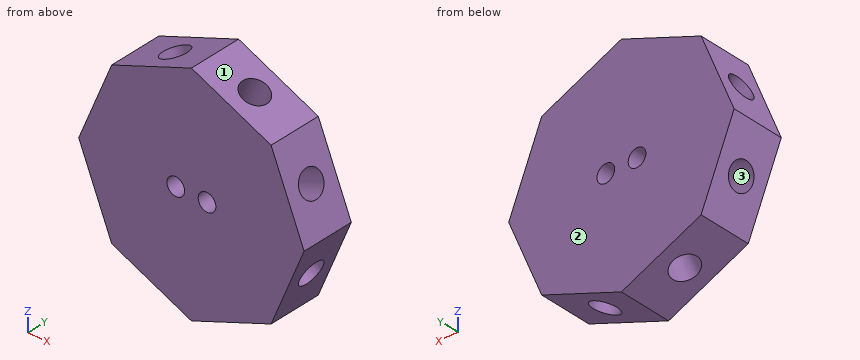
from build123d import *

# Parameters (mm, degrees)
SKETCH1_R           = 1.0795
BOSS_EXTRUDE1_DEPTH = 6.35
SKETCH2_R           = 1.5875
CUT_EXTRUDE1_DEPTH  = 7.62
CIRPATTERN1_COUNT   = 8


with BuildPart() as part:
    # Sketch1 → Boss-Extrude1 (new body)
    with BuildSketch(Plane(origin=(0, 0, 0), x_dir=(1, 0, 0), z_dir=(0, 1, 0))):
        Polygon((0, 13.746380944), (-9.720159182, 9.720159182), (-13.746380944, 0), (-9.720159182, -9.720159182), (0, -13.746380944), (9.720159182, -9.720159182), (13.746380944, 0), (9.720159182, 9.720159182), align=None)
        with Locations(Location((1.905, 0, 0), (0, 0, 270))):
            Circle(SKETCH1_R, mode=Mode.SUBTRACT)
        with Locations(Location((-1.905, 0, 0), (0, 0, 270))):
            Circle(SKETCH1_R, mode=Mode.SUBTRACT)
    extrude(amount=BOSS_EXTRUDE1_DEPTH)

    # Sketch2 → Cut-Extrude1 (cut)
    with BuildSketch(Plane(origin=(-4.860079591, 0, 11.733270063), x_dir=(0.9238795325112905, 0, 0.3826834323650806), z_dir=(-0.3826834323650806, 0, 0.9238795325112905))):
        with Locations((0, 3.175)):
            Circle(SKETCH2_R)
    cut_extrude1 = extrude(amount=-CUT_EXTRUDE1_DEPTH, mode=Mode.SUBTRACT)

    # CirPattern1: Cut-Extrude1 ×8 about axis
    cirpattern1_axis = Axis((0, 0, 0), (0, 1, 0))
    for i in range(1, CIRPATTERN1_COUNT):
        add(cut_extrude1.rotate(cirpattern1_axis, i * 360 / CIRPATTERN1_COUNT), mode=Mode.SUBTRACT)


solid = part.part
Verification items for the finished model (mm, model axes). Face numbers are marked on the shaded views. Coordinates: 2 decimals unless noted, no trailing zeros. Loops run counter-clockwise (first coordinate to the right, second up) from the corner with the lowest first, then second, coordinate; pieces in that order, holes last. Notation, with made-up numbers: (-28, -37.5) -> (13, -37.5) arc R22 cw to (13, -7.5) -> close; hole circle Ø6 at (39.25, -12.75). An arc over 180 degrees is marked (long way). Answer as a JSON object with one key per item and string values. Group by question number.
Item 1: Depth check by flat-ended pin: pin 1 (1 mm diameter, centred on x = 6.5, y = 3, fed in from -Z); pin 2 (3 mm diameter, centred on x = -1.905, z = 0, fed in from -Y); pin 3 (2 mm diameter, centred on x = 2, y = 1.5, fed in from -Z). Enter the tip coordinate at first touch or a pass-through.
Item 2: Mould release check, pull along Y, two halves, no side actions. Record for the marked faces 1, 2 and 3: +Y half, -Y half, draft (parallel to the pull), parting line (faces both ways), or undercut.
Item 3: Sectioned sample at B-B on x = -1.25. State how many separate pieces and enclosed holes the cut face has, plus the area to 3 significant figures.
Item 4: Sectioned sample at A-A on y = 5.5. Record the boundary of the cut face in (x, z) (1 decimal), plus the area to 3 significant figures.
Item 5: Scan lines: probe 1 along X at (y, z) = (1.75, 0); probe 2 along Z at (x, y) = (10.25, 2); probe 3 along X at (y, z) = (1.5, 0.5). Record each from-to range of solid material in increasing order.
Evaluation:
{
 "1": {"pin 1": "stops at z = -11.17", "pin 2": "stops at y = 0", "pin 3": "stops at z = -13.33"},
 "2": {"face 1": "draft", "face 2": "+Y half", "face 3": "undercut"},
 "3": {"separate pieces": "2", "enclosed holes": "2", "area": "148 mm²"},
 "4": {"outline": "(-13.7, 0) -> (-9.7, -9.7) -> (0, -13.7) -> (9.7, -9.7) -> (13.7, 0) -> (9.7, 9.7) -> (0, 13.7) -> (-9.7, 9.7) -> close; hole circle Ø2.2 at (-1.9, 0); hole circle Ø2.2 at (1.9, 0)", "area": "527 mm²"},
 "5": {"probe 1": "x = -13.75 to -2.98, -0.83 to 0.83, 2.98 to 13.75", "probe 2": "z = -8.44 to -5.4, -3.09 to 3.09, 5.4 to 8.44", "probe 3": "x = -13.54 to -2.86, -0.95 to 0.95, 2.86 to 13.54"}
}
